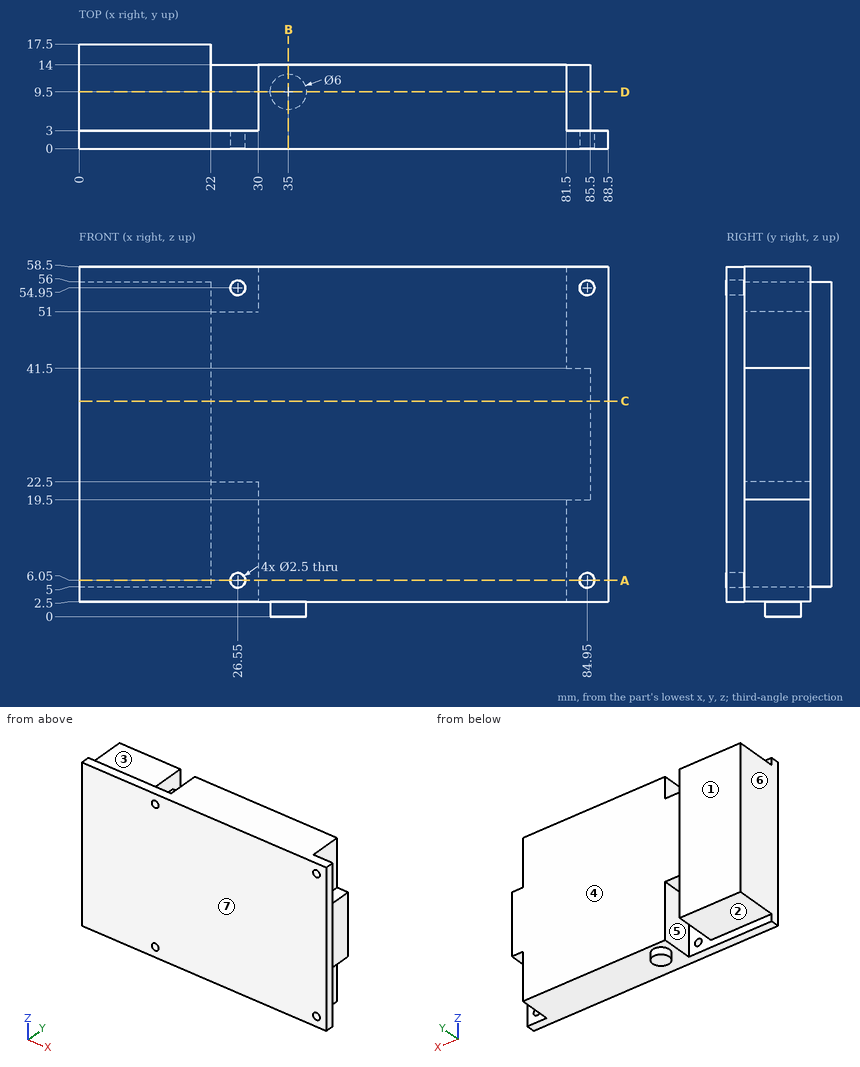
Could you check a few things on this drawing? It's one solid part, dimensions in mm from its lowest x, y, z. A direction names the side the tool comes from. Round coordinates to 2 decimals unless told otherwise and drop trailing zeros. Order: outer loops, then holes, each group sorted by start corner. A loop starts at its lowest first (then second) coordinate and runs counter-clockwise, first axis right, second up.
(1) Please list where these lines run through material, in increasing order: line 1 along X through (y, z) = (1.2, 54.95); line 2 along Z through (x, y) = (26.55, 1.7); line 3 along X through (y, z) = (6.5, 7).
Response values:
line 1: x = 0 to 25.3, 27.8 to 83.7, 86.2 to 88.5
line 2: z = 2.5 to 4.8, 7.3 to 53.7, 56.2 to 58.5
line 3: x = 0 to 22, 30 to 81.5
(2) I'm going to push flat-ended pins straight in: pin 1 (5.5 mm diameter, centred on x = 84.5, z = 18, fed in from +Y); pin 2 (2 mm diameter, centred on x = 84.95, z = 54.95, fed in from -Y); pin 3 (3 mm diameter, centred on x = 51.5, y = 9.5, fed in from -Z); pin 4 (9 mm diameter, centred on y = 9, z = 50.5, fed in from +X). Where does each tip first touch, or does it pass through?
Response values:
pin 1: stops at y = 14
pin 2: passes through
pin 3: stops at z = 2.5
pin 4: stops at x = 81.5
(3) Imagine slicing it at B-B (x = 35). Write out the boundary of the cut face in (y, z), plus the area to 3 significant figures.
Response values:
outline: (0, 2.5) - (6.5, 2.5) - (6.5, 0) - (12.5, 0) - (12.5, 2.5) - (14, 2.5) - (14, 58.5) - (0, 58.5) - close
area: 799 mm2
(4) Imagine slicing it at C-C (z = 36). Write out the boundary of the cut face in (x, y).
Response values:
outline: (0, 0) - (88.5, 0) - (88.5, 3) - (85.5, 3) - (85.5, 14) - (22, 14) - (22, 17.5) - (0, 17.5) - close
(5) If we mould it in two halves opening along X, with no side actions, what happens to the marked faces 5, 6 and 7? For each: released by +X, released by -X, zero draft, split by the parting line, or undercut.
Response values:
face 5: undercut
face 6: released by -X
face 7: zero draft
(6) Imagine slicing it at A-A (z = 6.05). Write out the boundary of the cut face in (x, y).
Response values:
outline: (0, 0) - (25.3, 0) - (25.3, 3) - (22, 3) - (22, 17.5) - (0, 17.5) - close; (27.8, 0) - (83.7, 0) - (83.7, 3) - (81.5, 3) - (81.5, 14) - (30, 14) - (30, 3) - (27.8, 3) - close; (86.2, 0) - (88.5, 0) - (88.5, 3) - (86.2, 3) - close
(7) Which directions (+Z, -Z, +X, -X, +Y, -Y) give clear straight access to the entire face, cutting with the end or side of a thin tool? Please do the marked faces 1, 2, 3 and 4.
Response values:
face 1: +Z, -Z, +X, -X, +Y
face 2: -Z, -X, +Y
face 3: +Z, -X, +Y
face 4: +Z, -Z, +X, +Y
(8) Imagine slicing it at D-D (y = 9.5). Write out the boundary of the cut face in (x, z).
Response values:
outline: (0, 5) - (22, 5) - (22, 22.5) - (30, 22.5) - (30, 2.5) - (32, 2.5) - (32, 0) - (38, 0) - (38, 2.5) - (81.5, 2.5) - (81.5, 19.5) - (85.5, 19.5) - (85.5, 41.5) - (81.5, 41.5) - (81.5, 58.5) - (30, 58.5) - (30, 51) - (22, 51) - (22, 56) - (0, 56) - close
